from build123d import *

# Parameters (mm, degrees)
F0_W     = 63.5
F0_H     = 38.1
F1_DEPTH = 25.4
F3_DEPTH = 25.401


with BuildPart() as f1:
    # F0 (on Front) → F1 (new body)
    with BuildSketch(Plane.XZ):
        with Locations((-31.75, 19.05)):
            Rectangle(F0_W, F0_H)
    extrude(amount=F1_DEPTH)

    # F2 (on face) → F3 (cut, through all)
    with BuildSketch(Plane.XZ.offset(25.4)):
        with BuildLine():
            Line((-12.7, 38.1), (-53.134321885, 38.1))
            ThreePointArc((-53.134321885, 38.1), (-32.9171609425, 19.0326653727), (-12.7, 38.1))
        make_face()
    extrude(amount=-F3_DEPTH, mode=Mode.SUBTRACT)


solid = f1.part
Design review of the part built by this model. Coordinates are the model's own, in mm. Round coordinates to 2 decimals unless told otherwise and drop trailing zeros. Order: outer loops, then holes, each group sorted by start corner. A loop starts at its lowest first (then second) coordinate and runs counter-clockwise, first axis right, second up.
1) Clearance check with flat-ended pins moving along their axes: pin 1 Ø1 at (x, y) = (-45.5, -3.5) entering from +Z; pin 2 Ø4 at (y, z) = (-4.5, 4.5) entering from +X. State where each tip first meets the part, or that it passes through.
The answers:
pin 1: stops at z = 23.83
pin 2: stops at x = 0
2) Consider section B-B (y = -1.25). State the section outline as (x, z) points, plus the area to 3 significant figures.
The answers:
outline: (-63.5, 0) - (0, 0) - (0, 38.1) - (-12.7, 38.1) arc R20.25 cw to (-53.13, 38.1) - (-63.5, 38.1) - close
area: 1,820 mm2
3) Consider section D-D (x = -23). State the section outline as (y, z) points, plus the area to 3 significant figures.
The answers:
outline: (-25.4, 0) - (0, 0) - (0, 21.63) - (-25.4, 21.63) - close
area: 549 mm2
4) Consider section A-A (z = 32.5). State the section outline as (x, y) points, plus the area to 3 significant figures.
The answers:
outline: (-63.5, -25.4) - (-52, -25.4) - (-52, 0) - (-63.5, 0) - close; (-13.84, -25.4) - (0, -25.4) - (0, 0) - (-13.84, 0) - close
area: 644 mm2
5) For L1, parallel to X at y = -19.5, z = 30; L2, parallel to X at y = -3.5, z = 26; L3, parallel to Z at x = -44, y = -6.5, list the stretches that pass through material, from the lowest coordinate up.
The answers:
L1: x = -63.5 to -50.92, -14.92 to 0
L2: x = -63.5 to -48.2, -17.63 to 0
L3: z = 0 to 22.33
6) Consider section C-C (z = 26.5). State the section outline as (x, y) points.
The answers:
outline: (-63.5, -25.4) - (-48.62, -25.4) - (-48.62, 0) - (-63.5, 0) - close; (-17.21, -25.4) - (0, -25.4) - (0, 0) - (-17.21, 0) - close
7) Draft analysis for pull direction X (two halves, no side actions). For faces 1 (the flat face through (-6, -13, 38.1)), 2 (the cylindrical face through (-33.346, -12.878, 19.037)), 3 (the flat face through (-63.5, -13, 19)), 4 (the flat face through (0, -13, 19)), state which applies: released by +X, released by -X, zero draft, split by the parting line, or undercut.
The answers:
face 1: zero draft
face 2: undercut
face 3: released by -X
face 4: released by +X
